```python
from build123d import *

# Parameters (mm, degrees)
SKETCH1_W               = 8
SKETCH1_H               = 8
BOSS_EXTRUDE1_DEPTH     = 3
CUT_EXTRUDE1_DEPTH      = 12.704699911
CUT_EXTRUDE1_DEPTH_BACK = 12.704699911
CUT_EXTRUDE2_DEPTH      = 11
SKETCH4_R               = 1.75
CUT_EXTRUDE3_DEPTH      = 0.4
SKETCH5_W               = 8
SKETCH5_H               = 1
BOSS_EXTRUDE2_DEPTH     = 2
FILLET1_R               = 4
CUT_EXTRUDE4_DEPTH      = 0.4
SKETCH7_W               = 1.384615385
SKETCH7_H               = 0.333333334
CUT_EXTRUDE5_DEPTH      = 0.55


with BuildPart() as part:
    # Sketch1 → Boss-Extrude1 (new body)
    with BuildSketch(Plane(origin=(0, 0, 0), x_dir=(1, 0, 0), z_dir=(0, 1, 0))):
        with Locations((4, 4)):
            Rectangle(SKETCH1_W, SKETCH1_H)
    extrude(amount=BOSS_EXTRUDE1_DEPTH)

    # Sketch2 → Cut-Extrude1 (cut, two sides: drawn at the far end of the back side and taken through both)
    with BuildSketch(Plane.XY.offset(-CUT_EXTRUDE1_DEPTH_BACK)):
        Polygon((0, 0), (0.6, 3), (0, 3), align=None)
        Polygon((8, 0), (7.4, 3), (8, 3), align=None)
    extrude(amount=CUT_EXTRUDE1_DEPTH + CUT_EXTRUDE1_DEPTH_BACK, mode=Mode.SUBTRACT)

    # Sketch3 → Cut-Extrude2 (cut)
    with BuildSketch(Plane(origin=(0, 0, 0), x_dir=(0, 0, -1), z_dir=(1, 0, 0))):
        Polygon((0, 0), (0.6, 3), (0, 3), align=None)
        Polygon((8, 3), (7.4, 3), (8, 0), align=None)
    extrude(amount=CUT_EXTRUDE2_DEPTH, mode=Mode.SUBTRACT)

    # Sketch4 → Cut-Extrude3 (cut)
    with BuildSketch(Plane.XZ):
        with Locations(Location((4, -3.75, 0), (0, 0, 270))):
            Circle(SKETCH4_R)
    extrude(amount=-CUT_EXTRUDE3_DEPTH, mode=Mode.SUBTRACT)

    # Sketch5 → Boss-Extrude2 (add)
    with BuildSketch(Plane.XZ):
        with Locations((4, -7.5)):
            Rectangle(SKETCH5_W, SKETCH5_H)
    extrude(amount=BOSS_EXTRUDE2_DEPTH)

    # Fillet1
    # the kernel refuses this fillet: 4 mm, written as the material it takes off along each edge
    with BuildSketch(Plane(origin=(8, -2, -16.660254038), x_dir=(0, 1, 0), z_dir=(0, 0, 1)), Plane(origin=(0, -2, 1.660254038), x_dir=(0, 1, 0), z_dir=(0, 0, -1))) as fillet1_piece_1:
        with BuildLine():
            CenterArc((4, 3.464101615), FILLET1_R, 180, 60)
            Line((0, 3.464101615), (-0.08, 3.464101615))
            Line((-0.08, 3.464101615), (-0.08, 0))
            Line((-0.08, 0), (0, -0.08))
            ThreePointArc((0, -0.08), (1, -0.08), (1.96, -0.069282032))
            Line((1.96, -0.069282032), (2, 0))
        make_face()
    extrude(amount=18.320508076, mode=Mode.SUBTRACT)

    # Sketch6 → Cut-Extrude4 (cut)
    with BuildSketch(Plane(origin=(0, 3, 0), x_dir=(1, 0, 0), z_dir=(0, 1, 0))):
        with BuildLine():
            Line((2.436272881, 5.979723732), (3.903420317, 5.979723732))
            add(Edge.make_bspline(
                [(3.903420317, 5.979723732), (3.943490496, 5.979744505), (4.021516441, 5.979784954), (4.134752515, 5.975087302), (4.240642802, 5.970362082), (4.338883372, 5.960903224), (4.429815049, 5.950988663), (4.51360101, 5.938436084), (4.589711972, 5.922348579), (4.637707501, 5.909661658), (4.660631856, 5.903601937)],
                knots=[0, 0, 0, 0, 1.259756885, 2.453039283, 3.563158368, 4.591894114, 5.55549294, 6.43918076, 7.254497783, 8, 8, 8, 8], degree=3))
            add(Edge.make_bspline(
                [(4.660631856, 5.903601937), (4.689300162, 5.894258489), (4.74612039, 5.87573989), (4.829420592, 5.843292221), (4.908343197, 5.803050568), (4.985816138, 5.760749105), (5.058380803, 5.710732544), (5.129877456, 5.658697008), (5.195666079, 5.598419283), (5.281939397, 5.514177193), (5.380383811, 5.396825298), (5.483519335, 5.241163905), (5.570813292, 5.070304112), (5.630456537, 4.917219685), (5.670729972, 4.787084992), (5.697056277, 4.682749965), (5.719418871, 4.572846322), (5.737778631, 4.457346355), (5.752043635, 4.336250048), (5.762664083, 4.209589679), (5.767837312, 4.07725583), (5.769008616, 3.987205692), (5.769606215, 3.941262194)],
                knots=[0, 0, 0, 0, 0.745524535, 1.477620414, 2.207090574, 2.934465325, 3.657932502, 4.384347339, 5.118673636, 5.861150177, 7.365375624, 8.894729774, 10.468936425, 12.099947606, 12.950091786, 13.83580991, 14.759228729, 15.722225242, 16.726454549, 17.773376212, 18.863978586, 20, 20, 20, 20], degree=3))
            add(Edge.make_bspline(
                [(5.769606215, 3.941262194), (5.768515323, 3.861857727), (5.766405561, 3.708291084), (5.741963835, 3.486695058), (5.70674022, 3.280872561), (5.667035899, 3.152471539), (5.647811343, 3.090300655)],
                knots=[0, 0, 0, 0, 1.103207939, 2.133582005, 3.096293362, 4, 4, 4, 4], degree=3))
            add(Edge.make_bspline(
                [(5.647811343, 3.090300655), (5.635116766, 3.054625647), (5.610144552, 2.98444734), (5.566445051, 2.883214788), (5.519227431, 2.786877042), (5.468100041, 2.695510004), (5.412804571, 2.609524646), (5.353134197, 2.529178156), (5.290013855, 2.453412746), (5.244286819, 2.406778778), (5.221529292, 2.383569886)],
                knots=[0, 0, 0, 0, 1.090884612, 2.145940218, 3.175104604, 4.181306866, 5.161203701, 6.118658341, 7.063689906, 8, 8, 8, 8], degree=3))
            add(Edge.make_bspline(
                [(5.221529292, 2.383569886), (5.184702113, 2.350450915), (5.108759222, 2.282154876), (4.974934842, 2.197635799), (4.823675662, 2.122952418), (4.714264019, 2.084588805), (4.657426727, 2.06465963)],
                knots=[0, 0, 0, 0, 0.908140292, 1.872714733, 2.8949153, 4, 4, 4, 4], degree=3))
            add(Edge.make_bspline(
                [(4.657426727, 2.06465963), (4.634546833, 2.057632533), (4.587060796, 2.043048157), (4.511767003, 2.027471741), (4.431388989, 2.011061834), (4.344999886, 2.001176252), (4.253496453, 1.990751469), (4.156149493, 1.984898536), (4.053296456, 1.980743294), (3.98275208, 1.980068625), (3.946689548, 1.979723732)],
                knots=[0, 0, 0, 0, 0.799129865, 1.658552685, 2.566799617, 3.538529252, 4.561352959, 5.643373779, 6.795284424, 8, 8, 8, 8], degree=3))
            Line((3.946689548, 1.979723732), (2.436272881, 1.979723732))
            Line((2.436272881, 1.979723732), (2.436272881, 5.979723732))
        make_face()
        with BuildLine():
            Line((3.205503651, 5.313057065), (3.205503651, 2.646390399))
            Line((3.205503651, 2.646390399), (3.838516471, 2.646390399))
            add(Edge.make_bspline(
                [(3.838516471, 2.646390399), (3.86709534, 2.646617049), (3.922120581, 2.647053436), (4.001743514, 2.648335709), (4.07491632, 2.651807064), (4.142022322, 2.655402822), (4.202886818, 2.661343643), (4.257774639, 2.667186667), (4.306380252, 2.675360935), (4.336400272, 2.681813595), (4.350535702, 2.684851937)],
                knots=[0, 0, 0, 0, 1.333384787, 2.567275092, 3.714769766, 4.750907381, 5.701951617, 6.567520054, 7.325492842, 8, 8, 8, 8], degree=3))
            add(Edge.make_bspline(
                [(4.350535702, 2.684851937), (4.38364248, 2.693686468), (4.44812575, 2.710893803), (4.538666782, 2.749253907), (4.62059475, 2.795531175), (4.695281698, 2.8511776), (4.762590099, 2.92150181), (4.820046047, 3.011440962), (4.873220012, 3.118706088), (4.909633556, 3.221385639), (4.935771128, 3.313096613), (4.95346412, 3.390071897), (4.967446413, 3.47335137), (4.979473009, 3.562606359), (4.989190784, 3.657722085), (4.995237644, 3.759042029), (4.999364663, 3.866442163), (5.000032135, 3.940189623), (5.000375445, 3.978121168)],
                knots=[0, 0, 0, 0, 1.038686998, 2.023088296, 2.974059649, 3.888265163, 4.839857954, 5.909819677, 7.113156087, 8.466843969, 9.20827164, 10.006482943, 10.861893492, 11.769681931, 12.739021491, 13.762258324, 14.849031541, 16, 16, 16, 16], degree=3))
            add(Edge.make_bspline(
                [(5.000375445, 3.978121168), (5.000034775, 4.01605283), (4.999374834, 4.089533605), (4.995254144, 4.196132914), (4.989241251, 4.29585735), (4.979454269, 4.38883019), (4.967614104, 4.475179926), (4.953468032, 4.554979633), (4.935881696, 4.627705609), (4.909721893, 4.71410541), (4.870064977, 4.811221472), (4.816099655, 4.917402921), (4.749828382, 5.00790436), (4.676605078, 5.08652444), (4.592177372, 5.151224792), (4.498716105, 5.205415106), (4.394186359, 5.247475499), (4.319831067, 5.2653904), (4.281625445, 5.274595527)],
                knots=[0, 0, 0, 0, 1.117996097, 2.165769068, 3.143980016, 4.062055362, 4.920439205, 5.712587309, 6.449616741, 7.124491204, 8.371470382, 9.537068822, 10.625202851, 11.666538334, 12.693249444, 13.747832046, 14.842779399, 16, 16, 16, 16], degree=3))
            add(Edge.make_bspline(
                [(4.281625445, 5.274595527), (4.265088191, 5.27766838), (4.228679487, 5.284433627), (4.168262747, 5.292335475), (4.097380449, 5.298199321), (4.015671249, 5.304185793), (3.923465993, 5.307602683), (3.820378875, 5.311168762), (3.706841263, 5.312386928), (3.627511913, 5.312827267), (3.586112625, 5.313057065)],
                knots=[0, 0, 0, 0, 0.578738571, 1.274160813, 2.095454135, 3.025967819, 4.093109015, 5.270126069, 6.575371698, 8, 8, 8, 8], degree=3))
            Line((3.586112625, 5.313057065), (3.205503651, 5.313057065))
        make_face(mode=Mode.SUBTRACT)
    extrude(amount=-CUT_EXTRUDE4_DEPTH, mode=Mode.SUBTRACT)

    # Sketch7 → Cut-Extrude5 (cut)
    with BuildSketch(Plane(origin=(0, 3, 0), x_dir=(1, 0, 0), z_dir=(0, 1, 0))):
        with Locations((6.167407218, 1.778686134)):
            Rectangle(SKETCH7_W, SKETCH7_H)
        with Locations((6.167407218, 1.188942544)):
            Rectangle(SKETCH7_W, SKETCH7_H)
    extrude(amount=-CUT_EXTRUDE5_DEPTH, mode=Mode.SUBTRACT)


solid = part.part
```
Read the model definition and answer for the solid it produces. Units are mm, in the model's axes. A direction names the side the tool comes from. Give positions to 0.01 mm unless a question says otherwise; leave off trailing zeros. Loops run counter-clockwise (first coordinate to the right, second up) from the corner with the lowest first, then second, coordinate; pieces in that order, holes last.
Item 1: Find the intervals of material crossed by line 1 along Y through (x, z) = (6, -2); line 2 along X through (y, z) = (0.3, -3.75); line 3 along X through (y, z) = (0.1, -3.75), in increasing order.
Item 2: The part is cut by section A-A (x = 1). Write down the section's boundary in (y, z), and give its area (3 significant figures).
Item 3: The mould has two halves that part along X. Classify faces 1 (the cylindrical face through (1.49, -1.48, -7.49)), 2 (the flat face through (3, 2.6, -4)), 3 (the flat face through (3, 0, -2)): released by +X, released by -X, zero draft, split by the parting line, or undercut.
Item 4: The part is cut by section B-B (z = -0.75). Write down the section's boundary in (x, y).
Item 5: The part is cut by section D-D (x = 6). Write down the section's boundary in (y, z), and give its area (3 significant figures).
Item 6: For faces 4 (the flat face through (4, -1, -7)), 5 (the flat face through (4, 0.4, -4)), 6 (the flat face through (0.3, 1.5, -4.1)), determine the directions among +Z, -Z, +X, -X, +Y, -Y from which every point of the face is accessible in a straight line to the end or side of a thin tool.
Item 7: Each of these flat-tipped pins is pushed along its axis until it touches: pin 1 Ø1.8 at (x, z) = (4.5, -3.5) entering from -Y; pin 2 Ø0.6 at (x, y) = (6.5, 2.5) entering from +Z; pin 3 Ø2 at (x, z) = (3.5, -2) entering from -Y. Where does it stop, or does it pass through?
Item 8: The part is cut by section C-C (y = 2.25). Write down the section's boundary in (x, z).
Taken from the geometry:
1. line 1: y = 0 to 3
1. line 2: x = 0.06 to 2.25, 5.75 to 7.94
1. line 3: x = 0.02 to 2.25, 5.75 to 7.98
2. outline: (-1.15, -8) - (0, -8) - (3, -7.4) - (3, -0.6) - (0, 0) - (0, -7) - (-1.15, -7) - close
2. area: 23.4 mm2
3. face 1: released by -X
3. face 2: undercut
3. face 3: zero draft
4. outline: (0, 0) - (8, 0) - (7.4, 3) - (0.6, 3) - close
5. outline: (-1.72, -8) - (0, -8) - (3, -7.4) - (3, -1.95) - (2.45, -1.95) - (2.45, -1.61) - (3, -1.61) - (3, -1.36) - (2.45, -1.36) - (2.45, -1.02) - (3, -1.02) - (3, -0.6) - (0, 0) - (0, -7) - (-1.72, -7) - close
5. area: 23.6 mm2
6. face 4: +Z, +X, -X, -Y
6. face 5: -Y
6. face 6: +Z, -Z, -X, +Y
7. pin 1: stops at y = 0.4
7. pin 2: stops at z = -0.44
7. pin 3: stops at y = 0
8. outline: (0.45, -7.55) - (7.55, -7.55) - (7.55, -0.45) - (0.45, -0.45) - close
